Build history of the part. All positions in model axes, mm. A direction names the side the tool comes from. Give positions to 0.01 mm unless a question says otherwise; leave off trailing zeros. Order: outer loops, then holes, each group sorted by start corner. A loop starts at its lowest first (then second) coordinate and runs counter-clockwise, first axis right, second up. Notation, with made-up numbers: (71.25, 80.25) - (108.25, 80.25) arc R34 ccw to (108.25, 118.25) - close; hole circle Ø3 at (89.5, 11). An arc over 180 degrees is marked (long way). One line per item, written item: value.
```python
from build123d import *

# Parameters (mm, degrees)
SKETCH2_R                    = 34
BOSS_EXTRUDE1_DEPTH          = 5
SKETCH3_R                    = 1.5
CUT_EXTRUDE1_DEPTH           = 5
SKETCH5_R                    = 1.5
CUT_EXTRUDE2_DEPTH           = 5
SKETCH6_R                    = 10
BOSS_EXTRUDE2_DEPTH          = 5
SKETCH7_R                    = 2
CUT_EXTRUDE3_DEPTH           = 5
SKETCH8_R                    = 3
CUT_EXTRUDE4_DEPTH           = 10
F_3_0_3_DIAMETER_HOLE1_D     = 3
F_3_0_3_DIAMETER_HOLE1_DEPTH = 7.84
F_3_0_3_DIAMETER_HOLE1_TIP   = 0.901290929


with BuildPart() as part:
    # Sketch2 → Boss-Extrude1 (new body)
    with BuildSketch(Plane(origin=(0, 0, 0), x_dir=(1, 0, 0), z_dir=(0, 1, 0))):
        with Locations(Location((0, 0, 0), (0, 0, 270))):
            Circle(SKETCH2_R)
    extrude(amount=BOSS_EXTRUDE1_DEPTH)

    # Sketch3 → Cut-Extrude1 (cut)
    with BuildSketch(Plane.XZ):
        with Locations(Location((0, 22, 0), (0, 0, 270))):
            Circle(SKETCH3_R)
        with Locations(Location((22, 0, 0), (0, 0, 270))):
            Circle(SKETCH3_R)
        with Locations(Location((0, -22, 0), (0, 0, 270))):
            Circle(SKETCH3_R)
        with Locations(Location((-22, 0, 0), (0, 0, 270))):
            Circle(SKETCH3_R)
    extrude(amount=-CUT_EXTRUDE1_DEPTH, mode=Mode.SUBTRACT)

    # Sketch5 → Cut-Extrude2 (cut)
    with BuildSketch(Plane.XZ):
        with Locations(Location((0, 15, 0), (0, 0, 270))):
            Circle(SKETCH5_R)
        with Locations(Location((15, 0, 0), (0, 0, 270))):
            Circle(SKETCH5_R)
        with Locations(Location((0, -15, 0), (0, 0, 270))):
            Circle(SKETCH5_R)
        with Locations(Location((-15, 0, 0), (0, 0, 270))):
            Circle(SKETCH5_R)
    extrude(amount=-CUT_EXTRUDE2_DEPTH, mode=Mode.SUBTRACT)

    # Sketch6 → Boss-Extrude2 (add)
    with BuildSketch(Plane.XZ):
        with Locations(Location((0, 0, 0), (0, 0, 270))):
            Circle(SKETCH6_R)
    extrude(amount=BOSS_EXTRUDE2_DEPTH)

    # Sketch7 → Cut-Extrude3 (cut)
    with BuildSketch(Plane(origin=(0, -5, 0), x_dir=(-1, 0, 0), z_dir=(0, -1, 0))):
        with Locations(Location((5.5, -3.985, 0), (0, 0, 90))):
            Circle(SKETCH7_R)
        with Locations(Location((-5.5, -3.985, 0), (0, 0, 270))):
            Circle(SKETCH7_R)
        with Locations(Location((-5.5, 3.985, 0), (0, 0, 90))):
            Circle(SKETCH7_R)
        with Locations(Location((5.5, 3.985, 0), (0, 0, 270))):
            Circle(SKETCH7_R)
    extrude(amount=-CUT_EXTRUDE3_DEPTH, mode=Mode.SUBTRACT)

    # Sketch8 → Cut-Extrude4 (cut)
    with BuildSketch(Plane.XZ.offset(5)):
        with Locations(Location((0, 0, 0), (0, 0, 270))):
            Circle(SKETCH8_R)
    extrude(amount=-CUT_EXTRUDE4_DEPTH, mode=Mode.SUBTRACT)

    # Ø3.0 (3) Diameter Hole1
    with Locations(Plane(origin=(0.026797027, -2.5, -9.999964096), x_dir=(-0.99999640959, 0, -0.002679702708), z_dir=(0.002679702708, 0, -0.99999640959))):
        with Locations((0, 0)):
            Hole(F_3_0_3_DIAMETER_HOLE1_D / 2, depth=F_3_0_3_DIAMETER_HOLE1_DEPTH)
            with Locations((0, 0, -(F_3_0_3_DIAMETER_HOLE1_DEPTH + F_3_0_3_DIAMETER_HOLE1_TIP / 2))):  # 118° drill point
                Cone(0, F_3_0_3_DIAMETER_HOLE1_D / 2, F_3_0_3_DIAMETER_HOLE1_TIP, mode=Mode.SUBTRACT)


solid = part.part
```
(1) Pin check, flat tips, straight feed: P1, Ø6, axis at x = -7.5, y = 2.5, coming from the +Z side; P2, Ø3, axis at y = 0, z = -7, coming from the +X side; P3, Ø2, axis at x = -11.5, z = 8, coming from the -Y side. Stop position of each tip, or through.
Completed:
P1: z = 33.7
P2: x = 33.55
P3: y = 0
(2) Slice it at D-D, the plane x = -4.5. Give the cut face in (y, z).
Completed:
outline: (-5, -8.93) - (0, -8.93) - (0, -33.7) - (5, -33.7) - (5, 33.7) - (0, 33.7) - (0, 8.93) - (-5, 8.93) - (-5, 5.72) - (0, 5.72) - (0, 2.25) - (-5, 2.25) - (-5, -2.25) - (0, -2.25) - (0, -5.72) - (-5, -5.72) - close
(3) Slice it at B-B, the plane x = 15. Give the cut face in (y, z), and give its area (3 significant figures).
Completed:
outline: (0, -30.51) - (5, -30.51) - (5, -1.5) - (0, -1.5) - close; (0, 1.5) - (5, 1.5) - (5, 30.51) - (0, 30.51) - close
area: 290 mm²
(4) Pull direction X, two halves, no side cores. Call faces 1 (the face through (-9.76, -2.46, 2.17)), 2 (the face through (8, 0, 7)), 3 (the face through (-5, 0, 4)): +X half, -X half, draft (parallel to the pull), parting line (faces both ways), or undercut.
Completed:
face 1: parting line
face 2: draft
face 3: undercut
(5) 3-axis set-ups, long thin cutter, end or side, ignore diameter. For faces 4 (the face through (6.101, -2.535, -5.893)), 5 (the face through (0.07, 2.46, -20.5)): which of +Z, -Z, +X, -X, +Y, -Y reach the whole face in a straight line?
Completed:
face 4: -Y
face 5: +Y, -Y
(6) Slice it at A-A, the plane y = 3.75. Count the separate pieces of the cut face and the enclosed holes in it, and give its area (3 significant figures).
Completed:
separate pieces: 1
enclosed holes: 9
area: 3,550 mm²
(7) Drill centre lines: line 1 (X direction, y = 1.15, z = 0); line 2 (X direction, y = 2.75, z = -0.5); line 3 (Y direction, x = 30, z = 5). Where is each one in solid material? Low to high.
Completed:
line 1: -34 to -23.5, -20.5 to -16.5, -13.5 to -3, 3 to 13.5, 16.5 to 20.5, 23.5 to 34
line 2: -34 to -23.41, -20.59 to -16.41, -13.59 to -2.96, 2.96 to 13.59, 16.41 to 20.59, 23.41 to 34
line 3: 0 to 5
(8) Slice it at C-C, the plane z = 22. Give the cut face in (x, y), and give its area (3 significant figures).
Completed:
outline: (-25.92, 0) - (-1.5, 0) - (-1.5, 5) - (-25.92, 5) - close; (1.5, 0) - (25.92, 0) - (25.92, 5) - (1.5, 5) - close
area: 244 mm²
